Geometry: final body of the model. Coordinates: model frame, mm. Give positions to 0.01 mm unless a question says otherwise; leave off trailing zeros. Write each loop counter-clockwise with the first axis right and the second up, starting at its lowest first coordinate (ties: lowest second). Pieces come first, ordered by that corner, then holes. Notation, with made-up numbers: (-4, 49.25) -> (23, 49.25) arc R25 cw to (23, 72.25) -> close; hole circle Ø8 at (72, 44.5). An arc over 180 degrees is marked (long way). Use CSV: the item, a comma, the result in double quotes. Start each with the question number.
1) Section C-C (z = 1.5). Output: boundary loops of the cut face in (x, y).
2) Section D-D (y = -16). Count the separate pieces of the cut face and the enclosed holes in it, plus the area to 3 significant figures.
3) Section B-B (y = 0). Output: boundary loops of the cut face in (x, z).
4) Material intervals for line 1 (Y direction, x = 0, z = 0.75); line 2 (X direction, y = -16.5, z = 0.9); line 3 (X direction, y = -13, z = 0.25), sorted ascending. Write a range as [from, to].
5) Contact query for a flat-ended pin moving along its axis: P1, Ø5, axis at x = 0, y = 32, coming from the +Z side. Output: stop coordinate, or through.
6) Section A-A (x = 0). Output: boundary loops of the cut face in (y, z).
7) Draft query along Y for faces 1 (the face through (-5, 26, 2)), 2 (the face through (28.775, -14.314, 0.986)), 3 (the face through (-4.686, 35.694, 0.296)). Return one class per face: pulls with the +Y half, pulls with the -Y half, needs draft (parallel to the pull), parting line crosses it, or undercut.
```python
from build123d import *

# Parameters (mm, degrees)
CYLINDER005_R     = 2
CYLINDER005_DEPTH = 10
CYLINDER006_R     = 2
CYLINDER006_DEPTH = 10
CYLINDER007_R     = 2
CYLINDER007_DEPTH = 10
CYLINDER001_R     = 26
CYLINDER001_DEPTH = 10
CYLINDER_R        = 36
CYLINDER_DEPTH    = 2
FILLET_R          = 1.4


with BuildPart() as cylinder005:
    # Cylinder005 → Cylinder005 (new body)
    with BuildSketch(Plane(origin=(0, 32, 0), x_dir=(1, 0, 0), z_dir=(0, 0, 1))):
        Circle(CYLINDER005_R)
    extrude(amount=CYLINDER005_DEPTH)


with BuildPart() as cylinder006:
    # Cylinder006 → Cylinder006 (new body)
    with BuildSketch(Plane(origin=(-27.7, -16, 0), x_dir=(1, 0, 0), z_dir=(0, 0, 1))):
        Circle(CYLINDER006_R)
    extrude(amount=CYLINDER006_DEPTH)


with BuildPart() as fusion:
    # Cylinder007 → Cylinder007 (new body)
    with BuildSketch(Plane(origin=(27.7, -16, 0), x_dir=(1, 0, 0), z_dir=(0, 0, 1))):
        Circle(CYLINDER007_R)
    extrude(amount=CYLINDER007_DEPTH)

    # Fusion: union Cylinder005, Cylinder006
    add(cylinder005.part)
    add(cylinder006.part)


with BuildPart() as cylinder001:
    # Cylinder001 → Cylinder001 (new body)
    with BuildSketch(Plane.XY):
        Circle(CYLINDER001_R)
    extrude(amount=CYLINDER001_DEPTH)


with BuildPart() as f_2in_ring:
    # Cylinder → Cylinder (new body)
    with BuildSketch(Plane.XY):
        Circle(CYLINDER_R)
    extrude(amount=CYLINDER_DEPTH)

    # Cut: cut Cylinder001
    add(cylinder001.part, mode=Mode.SUBTRACT)

    # Cut001: cut Fusion
    add(fusion.part, mode=Mode.SUBTRACT)

    # Fillet
    fillet_edges = [f_2in_ring.edges().sort_by_distance(p)[0] for p in [
        (-36, 0, 2),
    ]]
    fillet(fillet_edges, radius=FILLET_R)


solid = f_2in_ring.part
```
Answers follow:
1,outline,"circle Ø71.34 at (0, 0); hole circle Ø4 at (-27.7, -16); hole circle Ø52 at (0, 0); hole circle Ø4 at (0, 32); hole circle Ø4 at (27.7, -16)"
2,separate pieces,"4"
2,enclosed holes,"0"
2,area,"30.1 mm^2"
3,outline,"(-36, 0) -> (-26, 0) -> (-26, 2) -> (-34.6, 2) arc R1.4 ccw to (-36, 0.6) -> close; (26, 0) -> (36, 0) -> (36, 0.6) arc R1.4 ccw to (34.6, 2) -> (26, 2) -> close"
4,line 1,"y = [-35.99, -26], [26, 30], [34, 35.99]"
4,line 2,"x = [-31.96, -29.64], [-25.76, -20.09], [20.09, 25.76], [29.64, 31.96]"
4,line 3,"x = [-33.57, -22.52], [22.52, 33.57]"
5,P1,"stops at z = 2"
6,outline,"(-36, 0) -> (-26, 0) -> (-26, 2) -> (-34.6, 2) arc R1.4 ccw to (-36, 0.6) -> close; (26, 0) -> (30, 0) -> (30, 2) -> (26, 2) -> close; (34, 0) -> (36, 0) -> (36, 0.6) arc R1.4 ccw to (34.6, 2) -> (34, 2) -> close"
7,face 1,"needs draft"
7,face 2,"undercut"
7,face 3,"parting line crosses it"
